Design review of the part built by this model. Coordinates are the model's own, in mm. A direction names the side the tool comes from. Round coordinates to 2 decimals unless told otherwise and drop trailing zeros. Write each loop counter-clockwise with the first axis right and the second up, starting at its lowest first coordinate (ties: lowest second). Pieces come first, ordered by that corner, then holes. Notation, with made-up numbers: (54, 59) -> (61, 59) arc R26 cw to (61, 94) -> close; hole circle Ø2 at (62.5, 74.5). An arc over 180 degrees is marked (long way). One line per question, with ' | ' between items. Start each with the question number.
1) Consider section D-D (z = 6.25). Give the boundary of the cut face in (x, y), then the cut area to 3 significant figures.
2) Consider section C-C (z = 2). Give the boundary of the cut face in (x, y), then the cut area to 3 significant figures.
3) For faces 4 (the cylindrical face through (0, -1, 7)), 5 (the flat face through (0, 0, 9)), 6 (the flat face through (0, 0, 3)), list the 3-axis set-ups (+Z, -Z, +X, -X, +Y, -Y) from which the entire face can be reached by the end or side of a thin tool; tool diameter is ignored.
4) Consider section A-A (y = 0). Give the boundary of the cut face in (x, z).
5) For probe 1 along Y at (x, z) = (0, 1.9); probe 2 along Z at (x, y) = (-0.15, -0.25); probe 3 along Z at (x, y) = (0.6, 1.25), list the stretches that pass through material, from the lowest coordinate up.
6) Mouldability with a two-part tool opening along X and no side actions: class faces 1 (the cylindrical face through (-0.27, -1.22, 4.48)), 2 (the cylindrical face through (0.323, 0.506, 1.479)), 3 (the flat face through (1, 0, 0)) as +X half, -X half, draft (parallel to the pull), parting line (faces both ways), or undercut.
```python
from build123d import *

# Parameters (mm, degrees)
F1_R     = 1.25
F2_DEPTH = 6
F0_R     = 1
F3_DEPTH = 9
F4_R     = 1.5
F5_DEPTH = 3
F6_R     = 0.6
F7_DEPTH = 3


with BuildPart() as f2:
    # F1 (on Top) → F2 (new body)
    with BuildSketch(Plane.XY):
        Circle(F1_R)
    extrude(amount=F2_DEPTH)

    # F0 (on Top) → F3 (join)
    with BuildSketch(Plane.XY):
        Circle(F0_R)
    extrude(amount=F3_DEPTH)

    # F4 (on Top) → F5 (join)
    with BuildSketch(Plane.XY):
        Circle(F4_R)
    extrude(amount=F5_DEPTH)

    # F6 (on Top) → F7 (cut)
    with BuildSketch(Plane.XY):
        Circle(F6_R)
    extrude(amount=F7_DEPTH, mode=Mode.SUBTRACT)


solid = f2.part
```
From the geometry:
1) outline: circle Ø2 at (0, 0) | area: 3.14 mm2
2) outline: circle Ø3 at (0, 0); hole circle Ø1.2 at (0, 0) | area: 5.94 mm2
3) face 4: +Z | face 5: +Z, +X, -X, +Y, -Y | face 6: -Z
4) outline: (-1.5, 0) -> (-0.6, 0) -> (-0.6, 3) -> (0.6, 3) -> (0.6, 0) -> (1.5, 0) -> (1.5, 3) -> (1.25, 3) -> (1.25, 6) -> (1, 6) -> (1, 9) -> (-1, 9) -> (-1, 6) -> (-1.25, 6) -> (-1.25, 3) -> (-1.5, 3) -> close
5) probe 1: y = -1.5 to -0.6, 0.6 to 1.5 | probe 2: z = 3 to 9 | probe 3: z = 0 to 3
6) face 1: parting line | face 2: undercut | face 3: draft
